Work out the finished part from the listing and answer in its coordinate system (mm). Coordinates: 2 decimals unless noted, no trailing zeros. Order: outer loops, then holes, each group sorted by start corner. A loop starts at its lowest first (then second) coordinate and runs counter-clockwise, first axis right, second up.
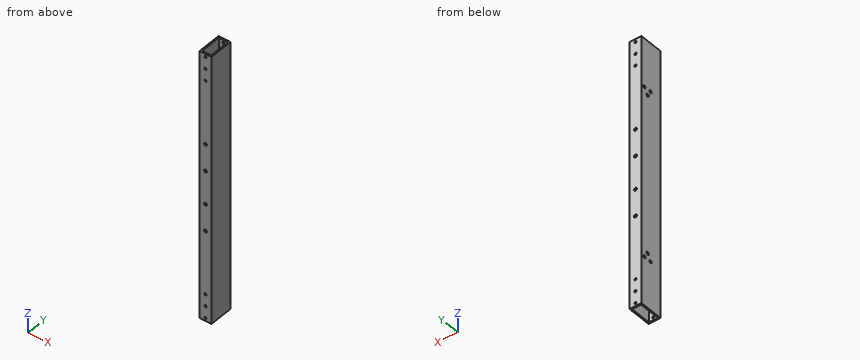
```python
from build123d import *

# Parameters (mm, degrees)
SKETCH1_W                      = 25.4
SKETCH1_H                      = 50.8
SKETCH1_W_2                    = 19.05
SKETCH1_H_2                    = 44.45
EXTRUDE_THIN1_DEPTH            = 571.5
F_3_16_0_1875_DIAMETER_HOLE1_D = 4.7625
F_1_4_0_25_DIAMETER_HOLE1_D    = 6.35
E_0_25_DIAMETER_HOLE1_D        = 6.35
E_0_25_DIAMETER_HOLE1_DEPTH    = 6.35
E_0_25_DIAMETER_HOLE1_TIP      = 1.907732465


with BuildPart() as part:
    # Sketch1 → Extrude-Thin1 (new body)
    with BuildSketch(Plane.XY):
        Rectangle(SKETCH1_W, SKETCH1_H)
        Rectangle(SKETCH1_W_2, SKETCH1_H_2, mode=Mode.SUBTRACT)
    extrude(amount=EXTRUDE_THIN1_DEPTH)

    # 3/16 (0.1875) Diameter Hole1 (through all)
    with Locations(Plane(origin=(0, 25.4, 565.15), x_dir=(0, 0, 1), z_dir=(0, 1, 0))):
        with Locations((0, 0), (-558.8, 0), (-533.4, 0), (-508, 0), (-25.4, 0), (-50.8, 0)):
            Hole(F_3_16_0_1875_DIAMETER_HOLE1_D / 2)

    # 1/4 (0.25) Diameter Hole1 (through all)
    with Locations(Plane(origin=(0, 25.4, 0), x_dir=(1, 0, 0), z_dir=(0, 1, 0))):
        with Locations((0, -321.183), (0, -378.333), (0, -192.786), (0, -249.936)):
            Hole(F_1_4_0_25_DIAMETER_HOLE1_D / 2)

    # E (0.25) Diameter Hole1
    with Locations(Plane.ZY.offset(12.7)):
        with Locations((103.886, 17.145), (103.886, 1.27), (116.586, 8.89), (454.914, 8.89), (467.614, 1.27), (467.614, 17.145)):
            Hole(E_0_25_DIAMETER_HOLE1_D / 2, depth=E_0_25_DIAMETER_HOLE1_DEPTH)
            with Locations((0, 0, -(E_0_25_DIAMETER_HOLE1_DEPTH + E_0_25_DIAMETER_HOLE1_TIP / 2))):  # 118° drill point
                Cone(0, E_0_25_DIAMETER_HOLE1_D / 2, E_0_25_DIAMETER_HOLE1_TIP, mode=Mode.SUBTRACT)


solid = part.part
```
1. The part is cut by section A-A (z = 76). Determine the outline of the cut face in (x, y) (3 decimals).
2. A flat-ended cylindrical pin translates along its axis: pin 1 (4 mm diameter, centred on y = 17.145, z = 103.886, fed in from -X) (3 decimals). Find the tip coordinate at first contact, or state that the pin passes through.
3. Consider probe 1 along Y at (x, z) = (-6.25, 228) (3 decimals); probe 2 along X at (y, z) = (-14.5, 200) (3 decimals); probe 3 along X at (y, z) = (22.95, 565.15). Determine where each line is inside the solid, lowest interval first.
Worked out:
1. outline: (-12.7, -25.4) - (12.7, -25.4) - (12.7, 25.4) - (-12.7, 25.4) - close; hole (-9.525, -22.225) - (9.525, -22.225) - (9.525, 22.225) - (-9.525, 22.225) - close
2. pin 1: stops at x = 9.525
3. probe 1: y = -25.4 to -22.225, 22.225 to 25.4
3. probe 2: x = -12.7 to -9.525, 9.525 to 12.7
3. probe 3: x = -12.7 to -2.38, 2.38 to 12.7
